CAD build for the part. Positions are in the model's coordinates, mm. Face numbers are marked on the shaded views. A direction names the side the tool comes from. Round coordinates to 2 decimals unless told otherwise and drop trailing zeros. Order: outer loops, then holes, each group sorted by start corner. A loop starts at its lowest first (then second) coordinate and runs counter-clockwise, first axis right, second up. Notation, with made-up numbers: M 6.5,63 L 10.5,63 A18 ccw 10.5,73 Z; hole C 18,2 d10. An arc over 180 degrees is marked long. Answer as a JSON object with one key per item and string values.
```python
from build123d import *

# Parameters (mm, degrees)
F1_DEPTH = 30
F2_W     = 24.6179879843
F2_H     = 6
F3_DEPTH = 42
F5_DEPTH = 24
F7_DEPTH = 100
F8_R     = 7.5
F9_DEPTH = 100


with BuildPart() as f1:
    # F0 (on Top) → F1 (new body)
    with BuildSketch(Plane.XY):
        with BuildLine():
            Line((-12.7826083564, 24.6179879843), (-30.7826083564, 24.6179879843))
            ThreePointArc((-30.7826083564, 24.6179879843), (-38.0569803183, 12.3089939921), (-30.7826083564, 0))
            Line((-30.7826083564, 0), (-12.7826083564, 0))
            Line((-12.7826083564, 0), (-12.7826083564, 24.6179879843))
        make_face()
    extrude(amount=F1_DEPTH)

    # F2 (on face) → F3 (join)
    with BuildSketch(Plane.YZ.offset(-12.7826083564)):
        with Locations((12.3089939921, 3)):
            Rectangle(F2_W, F2_H)
    extrude(amount=F3_DEPTH)

    # F4 (on face) → F5 (join)
    with BuildSketch(Plane.XY.offset(6)):
        Polygon((29.2173916436, 15.6179879843), (-12.7826083564, 15.8001863448), (-12.7826083564, 8.8001863448), (29.2173916436, 8.6179879843), align=None)
    extrude(amount=F5_DEPTH)

    # F6 (on face) → F7 (cut)
    with BuildSketch(Plane(origin=(0.0379344366, 8.7445701096, 0), x_dir=(0.9999905908, -0.0043380154, 0), z_dir=(-0.0043380154, -0.9999905908, 0))):
        Polygon((29.1797317659, 30), (-12.8206634256, 30), (29.1797317659, 6), align=None)
    extrude(amount=-F7_DEPTH, mode=Mode.SUBTRACT)

    # F8 (on face) → F9 (cut)
    with BuildSketch(Plane.XY.offset(30)):
        with Locations((-25.2924282104, 13.1551967934)):
            Circle(F8_R)
    extrude(amount=-F9_DEPTH, mode=Mode.SUBTRACT)


solid = f1.part
```
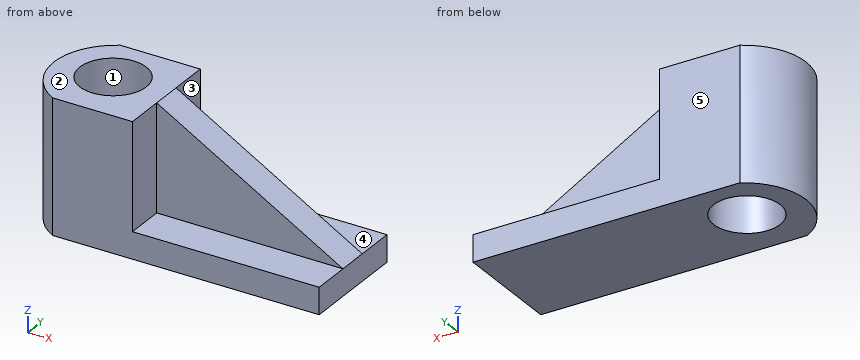
Item 1: Two-plate mould, pull along X, no slides. Class the marked faces 1, 2 and 3: released by +X, released by -X, zero draft, split by the parting line, or undercut.
Worked answers:
{"face 1": "undercut", "face 2": "zero draft", "face 3": "released by +X"}
Item 2: Saw through at B-B on y = 10.75. List the corners of the cut face in (x, z).
Worked answers:
{"outline": "M -37.97,0 L -32.4,0 L -32.4,30 L -37.97,30 Z; M -18.19,0 L 29.22,0 L 29.22,6.01 L -12.77,30 L -18.19,30 Z"}
Item 3: Saw through at C-C on x = -21.5. List the corners of the cut face in (y, z).
Worked answers:
{"outline": "M 0,0 L 6.68,0 L 6.68,30 L 0,30 Z; M 19.63,0 L 24.62,0 L 24.62,30 L 19.63,30 Z"}
Item 4: 3-axis set-ups, long thin cutter, end or side, ignore diameter. For the marked faces 4 and 5: which of +Z, -Z, +X, -X, +Y, -Y reach the whole face in a straight line?
Worked answers:
{"face 4": "+Z, +X, +Y", "face 5": "+Z, -Z, +X, -X, +Y"}
Item 5: Wall check: line 1 along Y through (x, z) = (-19.5, 12.5); line 2 along X through (y, z) = (8.5, 9.25); line 3 along Y through (x, z) = (-29, 11.5). Give the ranges that are in metal, low to high. Write a range as [from, to].
Worked answers:
{"line 1": "y = [0, 8.39], [17.92, 24.62]", "line 2": "x = [-37.53, -31.17], [-19.41, -12.78]", "line 3": "y = [0, 6.64], [19.67, 24.62]"}
Item 6: Saw through at D-D on z = 26.25. List the corners of the cut face in (x, y).
Worked answers:
{"outline": "M -30.78,0 L -12.78,0 L -12.78,8.8 L -6.22,8.77 L -6.19,15.77 L -12.78,15.8 L -12.78,24.62 L -30.78,24.62 A14.05 ccw Z; hole C -25.29,13.16 d15"}
Item 7: Drop flat-ended pins along their axis: pin 1 Ø10 at (x, y) = (18.5, 22) entering from +Z; pin 2 Ø1 at (y, z) = (5.5, 26) entering from +X; pin 3 Ø6 at (y, z) = (18, 10) entering from -X. Give the stop position or say it passes through.
Worked answers:
{"pin 1": "stops at z = 6", "pin 2": "stops at x = -12.78", "pin 3": "stops at x = -37.8"}
Item 8: Saw through at A-A on z = 9.75. List the corners of the cut face in (x, y).
Worked answers:
{"outline": "M -30.78,0 L -12.78,0 L -12.78,8.8 L 22.65,8.65 L 22.69,15.65 L -12.78,15.8 L -12.78,24.62 L -30.78,24.62 A14.05 ccw Z; hole C -25.29,13.16 d15"}
